Here's how the part is built. I have some questions about the finished solid (model axes, mm). Round coordinates to 2 decimals unless told otherwise and drop trailing zeros. Write each loop counter-clockwise with the first axis right and the second up, starting at its lowest first coordinate (ties: lowest second). Pieces come first, ordered by that corner, then holes. Notation, with made-up numbers: (48.25, -18.5) -> (97.25, -18.5) arc R21 cw to (97.25, 10.5) -> close; hole circle Ø4 at (3.5, -14.75). An arc over 180 degrees is marked (long way). Answer in a Markdown table with one row per item.
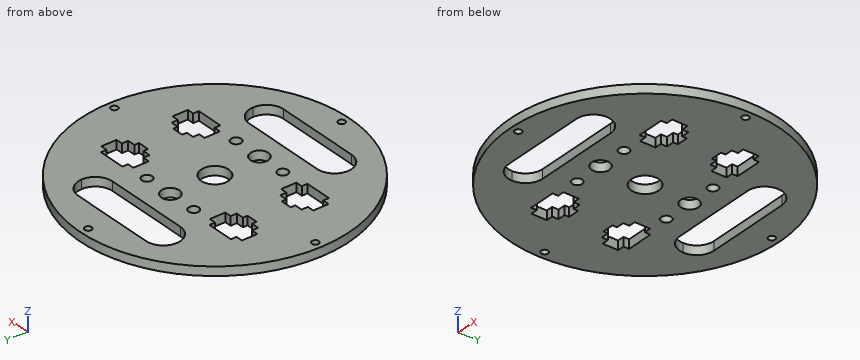
from build123d import *

# Parameters (mm, degrees)
SKETCH_1_R           = 50
EXTRUDE_1_DEPTH      = 3.302
SKETCH_4_R           = 5.08
CUT_EXTRUDE_3_DEPTH  = 71.787733429
SKETCH_7_R           = 1.27
CUT_EXTRUDE_6_DEPTH  = 71.787733429
SKETCH3_R            = 3.302
SKETCH3_R_2          = 1.9
CUT_EXTRUDE1_DEPTH   = 71.787733429
CUT_EXTRUDE4_DEPTH   = 71.787733429
MIRROR5_COPY_1_DEPTH = 71.787733429
SKETCH11_W           = 44.45
SKETCH11_H           = 12.7
CUT_EXTRUDE5_DEPTH   = 71.787733429
FILLET1_R            = 6.35
FILLET1_OF_MIRROR6_R = 6.35


with BuildPart() as part:
    # 草图1 → 凸台-拉伸1 (new body)
    with BuildSketch(Plane.XY):
        with Locations(Location((0, 0, 0), (0, 0, 180))):
            Circle(SKETCH_1_R)
    extrude(amount=EXTRUDE_1_DEPTH)

    # 草图4 → 切除-拉伸3 (cut, through all)
    with BuildSketch(Plane.XY.offset(3.302)):
        Circle(SKETCH_4_R)
    extrude(amount=-CUT_EXTRUDE_3_DEPTH, mode=Mode.SUBTRACT)

    # 草图7 → 切除-拉伸6 (cut, through all)
    with BuildSketch(Plane.XY.offset(3.302)):
        with Locations((0, 46.99)):
            Circle(SKETCH_7_R)
        with Locations((46.99, 0)):
            Circle(SKETCH_7_R)
        with Locations((0, -46.99)):
            Circle(SKETCH_7_R)
        with Locations((-46.99, 0)):
            Circle(SKETCH_7_R)
    extrude(amount=-CUT_EXTRUDE_6_DEPTH, mode=Mode.SUBTRACT)

    # Sketch3 → Cut-Extrude1 (cut, through all)
    with BuildSketch(Plane.XY.offset(3.302)):
        with Locations((0, 16.51)):
            Circle(SKETCH3_R)
        with Locations((10.922, 16.51)):
            Circle(SKETCH3_R_2)
        with Locations((-10.922, 16.51)):
            Circle(SKETCH3_R_2)
    cut_extrude1 = extrude(amount=-CUT_EXTRUDE1_DEPTH, mode=Mode.SUBTRACT)

    # Mirror3: Cut-Extrude1 across plane
    add(cut_extrude1.mirror(Plane.ZX), mode=Mode.SUBTRACT)

    # Sketch10 → Cut-Extrude4 (cut, through all)
    with BuildSketch(Plane.XY.offset(3.302)):
        Polygon((-20.4, -18.153199914), (-30.4, -18.153199914), (-30.4, -16.054784248), (-32.9, -16.054784248), (-32.9, -10.353195448), (-30.4, -10.353195448), (-30.4, -8.051599848), (-27.501596, -8.051599848), (-27.501596, -6.35), (-23.298404, -6.35), (-23.298404, -8.051599848), (-20.4, -8.051599848), (-20.4, -10.353195448), (-17.9, -10.353195448), (-17.9, -16.054784248), (-20.4, -16.054784248), align=None)
    cut_extrude4 = extrude(amount=-CUT_EXTRUDE4_DEPTH, mode=Mode.SUBTRACT)

    # Mirror4: Cut-Extrude4 across plane
    add(cut_extrude4.mirror(Plane.ZX), mode=Mode.SUBTRACT)

    # Mirror5: Cut-Extrude4 across plane
    add(cut_extrude4.mirror(Plane(origin=(0, 0, 0), x_dir=(0, 0, 1), z_dir=(1, 0, 0))), mode=Mode.SUBTRACT)

    # Mirror5 copy 1 sketch → Mirror5 copy 1 (cut, through all)
    with BuildSketch(Plane(origin=(0, 0, 3.302), x_dir=(-1, 0, 0), z_dir=(0, 0, 1))):
        Polygon((-20.4, -18.153199914), (-30.4, -18.153199914), (-30.4, -16.054784248), (-32.9, -16.054784248), (-32.9, -10.353195448), (-30.4, -10.353195448), (-30.4, -8.051599848), (-27.501596, -8.051599848), (-27.501596, -6.35), (-23.298404, -6.35), (-23.298404, -8.051599848), (-20.4, -8.051599848), (-20.4, -10.353195448), (-17.9, -10.353195448), (-17.9, -16.054784248), (-20.4, -16.054784248), align=None)
    extrude(amount=-MIRROR5_COPY_1_DEPTH, mode=Mode.SUBTRACT)

    # Sketch11 → Cut-Extrude5 (cut, through all)
    with BuildSketch(Plane.XY.offset(3.302)):
        with Locations((0, 31.75)):
            Rectangle(SKETCH11_W, SKETCH11_H)
    cut_extrude5 = extrude(amount=-CUT_EXTRUDE5_DEPTH, mode=Mode.SUBTRACT)

    # Fillet1
    fillet1_edges = [part.edges().sort_by_distance(p)[0] for p in [
        (22.225, 25.4, 1.651),
        (22.225, 38.1, 1.651),
        (-22.225, 38.1, 1.651),
        (-22.225, 25.4, 1.651),
    ]]
    fillet(fillet1_edges, radius=FILLET1_R - 0.0001)  # a hair under: the kernel refuses the full size

    # Mirror6: Cut-Extrude5 across plane
    add(cut_extrude5.mirror(Plane.ZX), mode=Mode.SUBTRACT)

    # Fillet1 of Mirror6
    fillet1_of_mirror6_edges = [part.edges().sort_by_distance(p)[0] for p in [
        (22.225, -25.4, 1.651),
        (22.225, -38.1, 1.651),
        (-22.225, -38.1, 1.651),
        (-22.225, -25.4, 1.651),
    ]]
    fillet(fillet1_of_mirror6_edges, radius=FILLET1_OF_MIRROR6_R - 0.0001)  # a hair under: the kernel refuses the full size


solid = part.part
1) I want a section at C-C, the plane y = 46.99. List the corners of the cut face in (x, z) for me, and give its area (3 significant figures).
Response:
| item | result |
|---|---|
| outline | (-17.09, 0) -> (-1.27, 0) -> (-1.27, 3.3) -> (-17.09, 3.3) -> close; (1.27, 0) -> (17.09, 0) -> (17.09, 3.3) -> (1.27, 3.3) -> close |
| area | 104 mm^2 |
2) For pin 1 (1.5 mm diameter, centred on x = 20.5, z = 0.5, fed in from +Y); pin 2 (1.7 mm diameter, centred on x = 25, z = 1.5, fed in from +Y); pin 3 (1.2 mm diameter, centred on x = -32, z = 2, fed in from +Y), each with a flat end and sliding along its axis, tell me the tip position at first contact or that it passes through.
Response:
| item | result |
|---|---|
| pin 1 | stops at y = 45.93 |
| pin 2 | stops at y = 43.78 |
| pin 3 | stops at y = 38.91 |
3) I want a section at A-A, the plane y = 0. List the corners of the cut face in (x, z) for me.
Response:
| item | result |
|---|---|
| outline | (-50, 0) -> (-48.26, 0) -> (-48.26, 3.3) -> (-50, 3.3) -> close; (-45.72, 0) -> (-5.08, 0) -> (-5.08, 3.3) -> (-45.72, 3.3) -> close; (5.08, 0) -> (45.72, 0) -> (45.72, 3.3) -> (5.08, 3.3) -> close; (48.26, 0) -> (50, 0) -> (50, 3.3) -> (48.26, 3.3) -> close |
4) I want a section at B-B, the plane x = 0. Count the separate pieces of the cut face and the enclosed holes in it, and give its area (3 significant figures).
Response:
| item | result |
|---|---|
| separate pieces | 8 |
| enclosed holes | 0 |
| area | 152 mm^2 |
5) I need wall thicknesses on line 1 (X direction, y = -16.51, z = 1.65); line 2 (Y direction, x = -27, z = 1.1); line 3 (Y direction, x = -18.5, z = 0.9). Which ranges of each line are inside material? Lowest first, please. Write a range as [from, to].
Response:
| item | result |
|---|---|
| line 1 | x = [-47.2, -30.4], [-20.4, -12.82], [-9.02, -3.3], [3.3, 9.02], [12.82, 20.4], [30.4, 47.2] |
| line 2 | y = [-42.08, -18.15], [-6.35, 6.35], [18.15, 42.08] |
| line 3 | y = [-46.45, -37.53], [-25.97, -16.05], [-10.35, 10.35], [16.05, 25.97], [37.53, 46.45] |
